Could you check a few things on this model? Use its own coordinates, in mm. A direction names the side the tool comes from. Coordinates: 2 decimals unless noted, no trailing zeros. Loops run counter-clockwise (first coordinate to the right, second up) from the corner with the lowest first, then second, coordinate; pieces in that order, holes last. Notation, with made-up numbers: (87, 17) -> (126, 17) arc R21 ccw to (126, 40) -> close; hole circle Ø1 at (47, 78.25). An arc over 180 degrees is marked (long way). One line per question, with ' | ' between items.
from build123d import *

# Parameters (mm, degrees)
SKETCH1_W           = 30
SKETCH1_H           = 10
SKETCH1_R           = 2.5
BOSS_EXTRUDE1_DEPTH = 2.5
SKETCH2_W           = 30
SKETCH2_H           = 2.5
BOSS_EXTRUDE2_DEPTH = 22.5
FILLET1_R           = 2


with BuildPart() as part:
    # Sketch1 → Boss-Extrude1 (new body)
    with BuildSketch(Plane(origin=(0, 0, 0), x_dir=(-1, 0, 0), z_dir=(0, 0, 1))):
        with Locations((-41.638953423, 46.1)):
            Rectangle(SKETCH1_W, SKETCH1_H)
        with Locations(Location((-49.138953423, 46.1, 0), (0, 0, 180))):
            Circle(SKETCH1_R, mode=Mode.SUBTRACT)
        with Locations((-34.138953423, 46.1)):
            Circle(SKETCH1_R, mode=Mode.SUBTRACT)
    extrude(amount=BOSS_EXTRUDE1_DEPTH)

    # Sketch2 → Boss-Extrude2 (add)
    with BuildSketch(Plane(origin=(0, 0, 0), x_dir=(-1, 0, 0), z_dir=(0, 0, -1))):
        with Locations((-41.638953423, -39.85)):
            Rectangle(SKETCH2_W, SKETCH2_H)
    extrude(amount=-BOSS_EXTRUDE2_DEPTH)

    # Fillet1
    fillet1_edges = [part.edges().sort_by_distance(p)[0] for p in [
        (26.638953423, -46.1, 2.5),
        (41.638953423, -51.1, 2.5),
        (41.638953423, -41.1, 22.5),
        (26.638953423, -41.1, 12.5),
        (26.638953423, -39.85, 22.5),
        (56.638953423, -39.85, 22.5),
        (56.638953423, -41.1, 12.5),
        (56.638953423, -46.1, 2.5),
        (56.638953423, -51.1, 1.25),
        (26.638953423, -51.1, 1.25),
        (41.638953423, -41.1, 2.5),
    ]]
    fillet(fillet1_edges, radius=FILLET1_R)


solid = part.part
1) If we section it at C-C on z = 18: Please give me the cut outline in (x, y), and give its area (3 significant figures).
Data:
outline: (26.64, -39.1) arc R2 ccw to (28.64, -41.1) -> (54.64, -41.1) arc R2 ccw to (56.64, -39.1) -> (56.64, -38.6) -> (26.64, -38.6) -> close | area: 73.3 mm²
2) On a 3-axis mill with a long thin cutter (end or side, diameter ignored), from which of +Z, -Z, +X, -X, +Y, -Y can I reach the whole of each face in a straight line? I mean faces 4 (the face through (27.21, -50.5, 0.25)), 5 (the face through (27.21, -40.5, 12.61)), 6 (the face through (56.07, -40.5, 12.61)). Say none if no direction works.
Data:
face 4: +Z, -Z, -X, -Y | face 5: +Z, -X, -Y | face 6: +Z, +X, -Y
3) If we section it at B-B on x = 39.5: Please give me the cut outline in (y, z).
Data:
outline: (-51.1, 0) -> (-38.6, 0) -> (-38.6, 22.5) -> (-39.1, 22.5) arc R2 ccw to (-41.1, 20.5) -> (-41.1, 4.5) arc R2 cw to (-43.1, 2.5) -> (-49.1, 2.5) arc R2 ccw to (-51.1, 0.5) -> close
4) If we section it at D-D on y = -50: Please give me the cut outline in (x, z), and give its area (3 significant figures).
Data:
outline: (26.85, 0) -> (56.43, 0) -> (56.43, 0.5) arc R1.79 ccw to (54.64, 2.29) -> (28.64, 2.29) arc R1.79 ccw to (26.85, 0.5) -> close | area: 66.2 mm²
5) I'm going to push flat-ended pins straight in: pin 1 Ø13 at (x, z) = (41, 13.5) entering from -Y; pin 2 Ø3 at (x, y) = (49.5, -41) entering from -Z; pin 3 Ø1.8 at (x, y) = (45, -44.5) entering from +Z. Where does each tip first touch, or does it pass through?
Data:
pin 1: y = -41.1 | pin 2: z = 0 | pin 3: z = 2.5
6) If we section it at A-A on y = -46.1: Please give me the cut outline in (x, z), and give its area (3 significant figures).
Data:
outline: (26.64, 0) -> (31.64, 0) -> (31.64, 2.5) -> (28.64, 2.5) arc R2 ccw to (26.64, 0.5) -> close; (36.64, 0) -> (46.64, 0) -> (46.64, 2.5) -> (36.64, 2.5) -> close; (51.64, 0) -> (56.64, 0) -> (56.64, 0.5) arc R2 ccw to (54.64, 2.5) -> (51.64, 2.5) -> close | area: 48.3 mm²
7) I need wall thicknesses on line 1 along Y through (x, z) = (35, 4.5); line 2 along Z through (x, y) = (54.75, -48); line 3 along Z through (x, y) = (53.5, -39.75). Which ranges of each line are inside material? Lowest first, please. Write a range as from..to.
Data:
line 1: -41.1..-38.6 | line 2: 0..2.5 | line 3: 0..22.39
8) We'd pull the mould along X, two halves only. Please class faces 1 (the face through (42, -41.1, 12)), 2 (the face through (34.68, -43.66, 1.23)), 3 (the face through (56.07, -50.5, 0.25)): pulls with the +X half, pulls with the -X half, needs draft (parallel to the pull), parting line crosses it, or undercut.
Data:
face 1: needs draft | face 2: undercut | face 3: pulls with the +X half
